from build123d import *

# Parameters (mm, degrees)
EXTRUDE_1_DEPTH     = 2
EXTRUDE_3_DEPTH     = 9
EXTRUDE_5_DEPTH     = 7
SKETCH_3_R          = 2.5
SKETCH_3_R_2        = 1.5
EXTRUDE_8_DEPTH     = 5
EXTRUDE_9_DEPTH     = 7
CUT_EXTRUDE_2_DEPTH = 5


with BuildPart() as part:
    # Sketch 1 → Extrude 1 (new body)
    with BuildSketch(Plane(origin=(0, 0, 0), x_dir=(1, 0, 0), z_dir=(0, 1, 0))):
        with BuildLine():
            Line((0, 28), (0, 40))
            ThreePointArc((0, 40), (10, 50), (20, 40))
            Line((20, 40), (20, 28))
            ThreePointArc((20, 28), (31.75, 29), (43.5, 28))
            Line((43.5, 28), (43.5, 40))
            ThreePointArc((43.5, 40), (53.5, 50), (63.5, 40))
            Line((63.5, 40), (63.5, 28))
            Line((63.5, 28), (63.5, 10))
            ThreePointArc((63.5, 10), (60.571067812, 2.928932188), (53.5, 0))
            Line((53.5, 0), (10, 0))
            ThreePointArc((10, 0), (2.928932188, 2.928932188), (0, 10))
            Line((0, 10), (0, 28))
        make_face()
    extrude(amount=EXTRUDE_1_DEPTH)

    # Sketch 1_4 → Extrude 3 (add)
    with BuildSketch(Plane(origin=(0, 0, 0), x_dir=(1, 0, 0), z_dir=(0, 1, 0))):
        with BuildLine():
            Line((42.5, 40), (42.5, 29.175957135))
            ThreePointArc((42.5, 29.175957135), (31.75, 30), (21, 29.175957135))
            Line((21, 29.175957135), (21, 40))
            ThreePointArc((21, 40), (10, 51), (-1, 40))
            Line((-1, 40), (-1, 28))
            Line((-1, 28), (-1, 10))
            ThreePointArc((-1, 10), (2.221825407, 2.221825407), (10, -1))
            Line((10, -1), (53.5, -1))
            ThreePointArc((53.5, -1), (61.278174593, 2.221825407), (64.5, 10))
            Line((64.5, 10), (64.5, 28))
            Line((64.5, 28), (64.5, 40))
            ThreePointArc((64.5, 40), (53.5, 51), (42.5, 40))
        make_face()
        with BuildLine():
            Line((0, 28), (0, 40))
            ThreePointArc((0, 40), (10, 50), (20, 40))
            Line((20, 40), (20, 28))
            ThreePointArc((20, 28), (31.75, 29), (43.5, 28))
            Line((43.5, 28), (43.5, 40))
            ThreePointArc((43.5, 40), (53.5, 50), (63.5, 40))
            Line((63.5, 40), (63.5, 28))
            Line((63.5, 28), (63.5, 10))
            ThreePointArc((63.5, 10), (60.571067812, 2.928932188), (53.5, 0))
            Line((53.5, 0), (10, 0))
            ThreePointArc((10, 0), (2.928932188, 2.928932188), (0, 10))
            Line((0, 10), (0, 28))
        make_face(mode=Mode.SUBTRACT)
    extrude(amount=EXTRUDE_3_DEPTH)

    # Sketch 1_6 → Extrude 5 (add)
    with BuildSketch(Plane(origin=(0, 0, 0), x_dir=(1, 0, 0), z_dir=(0, 1, 0))):
        with BuildLine():
            Line((10, -2), (53.5, -2))
            ThreePointArc((53.5, -2), (61.985281374, 1.514718626), (65.5, 10))
            Line((65.5, 10), (65.5, 28))
            Line((65.5, 28), (65.5, 40))
            ThreePointArc((65.5, 40), (53.5, 52), (41.5, 40))
            Line((41.5, 40), (41.5, 30.332402365))
            ThreePointArc((41.5, 30.332402365), (31.75, 31), (22, 30.332402365))
            Line((22, 30.332402365), (22, 40))
            ThreePointArc((22, 40), (10, 52), (-2, 40))
            Line((-2, 40), (-2, 28))
            Line((-2, 28), (-2, 10))
            ThreePointArc((-2, 10), (1.514718626, 1.514718626), (10, -2))
        make_face()
        with BuildLine():
            Line((42.5, 40), (42.5, 29.175957135))
            ThreePointArc((42.5, 29.175957135), (31.75, 30), (21, 29.175957135))
            Line((21, 29.175957135), (21, 40))
            ThreePointArc((21, 40), (10, 51), (-1, 40))
            Line((-1, 40), (-1, 28))
            Line((-1, 28), (-1, 10))
            ThreePointArc((-1, 10), (2.221825407, 2.221825407), (10, -1))
            Line((10, -1), (53.5, -1))
            ThreePointArc((53.5, -1), (61.278174593, 2.221825407), (64.5, 10))
            Line((64.5, 10), (64.5, 28))
            Line((64.5, 28), (64.5, 40))
            ThreePointArc((64.5, 40), (53.5, 51), (42.5, 40))
        make_face(mode=Mode.SUBTRACT)
    extrude(amount=EXTRUDE_5_DEPTH)

    # Sketch 3 → Extrude 8 (add)
    with BuildSketch(Plane(origin=(0, 2, 0), x_dir=(1, 0, 0), z_dir=(0, 1, 0))):
        with Locations((24.5, 24)):
            Circle(SKETCH_3_R)
        with Locations((24.5, 24)):
            Circle(SKETCH_3_R_2, mode=Mode.SUBTRACT)
        with Locations((42, 4)):
            Circle(SKETCH_3_R)
        with Locations((42, 4)):
            Circle(SKETCH_3_R_2, mode=Mode.SUBTRACT)
    extrude(amount=EXTRUDE_8_DEPTH)

    # Sketch 3_7 → Extrude 9 (add)
    with BuildSketch(Plane(origin=(0, 2, 0), x_dir=(1, 0, 0), z_dir=(0, 1, 0))):
        with BuildLine():
            Line((63.5, 13.5), (63.5, 16.5))
            ThreePointArc((63.5, 16.5), (62, 15), (63.5, 13.5))
        make_face()
        with BuildLine():
            Line((0, 16.5), (0, 13.5))
            ThreePointArc((0, 13.5), (1.5, 15), (0, 16.5))
        make_face()
        with BuildLine():
            ThreePointArc((36.25, 0), (33.25, 3), (30.25, 0))
            Line((30.25, 0), (36.25, 0))
        make_face()
    extrude(amount=EXTRUDE_9_DEPTH)

    # Sketch 4 → Cut-Extrude 2 (cut)
    with BuildSketch(Plane.ZY.offset(2)):
        with BuildLine():
            Line((-10, 4.5), (-10, 9))
            Line((-10, 9), (-5, 9))
            Line((-5, 9), (-5, 4.5))
            ThreePointArc((-5, 4.5), (-7.5, 2), (-10, 4.5))
        make_face()
    extrude(amount=-CUT_EXTRUDE_2_DEPTH, mode=Mode.SUBTRACT)


solid = part.part
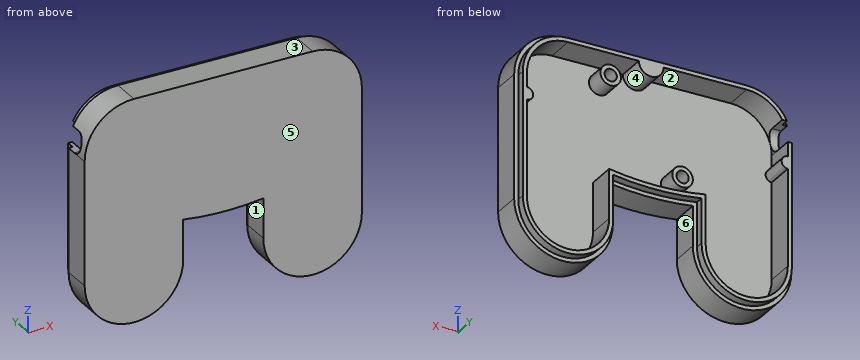
Design review of the part built by this model. Coordinates are the model's own, in mm. Face numbers are marked on the shaded views. A direction names the side the tool comes from. Round coordinates to 2 decimals unless told otherwise and drop trailing zeros. Loops run counter-clockwise (first coordinate to the right, second up) from the corner with the lowest first, then second, coordinate; pieces in that order, holes last. Notation, with made-up numbers: (-11, -16.5) - (33, -16.5) arc R24 ccw to (33, 10.5) - close; hole circle Ø10 at (74.25, 75). An arc over 180 degrees is marked (long way). One line per item, written item: value. Start each with the question number.
1) Consider section D-D on z = -24. Give the boundary of the cut face in (x, y), then the cut area to 3 significant figures.
2) To check wall thickness, follow L1, parallel to X at y = 3, z = -34.5; L2, parallel to X at y = 6, z = -22; L3, parallel to X at y = 4.4, z = -24. State the ranges of each line that lie inside material, in increasing order. Write a range as from..to.
3) Draft analysis for pull direction Z (two halves, no side actions). For the marked faces 1, 2 and 3, state which applies: +Z half, -Z half, draft (parallel to the pull), parting line (faces both ways), or undercut.
4) Insertion check: pin 1 Ø4 at (x, z) = (25.5, -24) entering from +Y; pin 2 Ø1.6 at (x, y) = (36.5, 8.5) entering from +Z; pin 3 Ø10 at (x, z) = (41.5, -12) entering from +Y. Each pin has a flat end and moves straight along its axis. Give the tip position at first contact, or say it passes through.
5) For the marked faces 4, 5 and 6, list the 3-axis set-ups (+Z, -Z, +X, -X, +Y, -Y) from which the entire face can be reached by the end or side of a thin tool; tool diameter is ignored.
6) Consider section B-B on y = 2.75. Give the number of separate pieces and of enclosed holes in the cut face, then the cut area to 3 significant figures.
7) Consider section A-A on z = -38. Give the boundary of the cut face in (x, y).
8) Consider section C-C on x = 6. Give the boundary of the cut face in (y, z), then the cut area to 3 significant figures.
Reported:
1. outline: (-2, 0) - (65.5, 0) - (65.5, 7) - (64.5, 7) - (64.5, 9) - (63.5, 9) - (63.5, 2) - (27, 2) - (27, 7) - (26, 7) - (26, 2) - (23, 2) - (23, 7) - (22, 7) - (22, 2) - (0, 2) - (0, 9) - (-1, 9) - (-1, 7) - (-2, 7) - close
1. area: 169 mm^2
2. L1: x = -2..0, 20..22, 41.5..43.5, 63.5..65.5
2. L2: x = -2..0, 23..26, 63.5..65.5
2. L3: x = -2..0, 22..23, 26..27, 63.5..65.5
3. face 1: draft
3. face 2: undercut
3. face 3: +Z half
4. pin 1: stops at y = 7
4. pin 2: stops at z = 1
4. pin 3: stops at y = 2
5. face 4: +Y
5. face 5: +Z, -Z, +X, -X, -Y
5. face 6: -Z, +Y, -Y
6. separate pieces: 3
6. enclosed holes: 2
6. area: 540 mm^2
7. outline: (-2, 0) - (22, 0) - (22, 7) - (21, 7) - (21, 9) - (20, 9) - (20, 2) - (0, 2) - (0, 9) - (-1, 9) - (-1, 7) - (-2, 7) - close; (41.5, 0) - (65.5, 0) - (65.5, 7) - (64.5, 7) - (64.5, 9) - (63.5, 9) - (63.5, 2) - (43.5, 2) - (43.5, 9) - (42.5, 9) - (42.5, 7) - (41.5, 7) - close
8. outline: (0, -51.31) - (7, -51.31) - (7, -50.25) - (9, -50.25) - (9, -49.17) - (2, -49.17) - (2, -0.83) - (9, -0.83) - (9, 0.25) - (7, 0.25) - (7, 1.31) - (0, 1.31) - close
8. area: 131 mm^2
